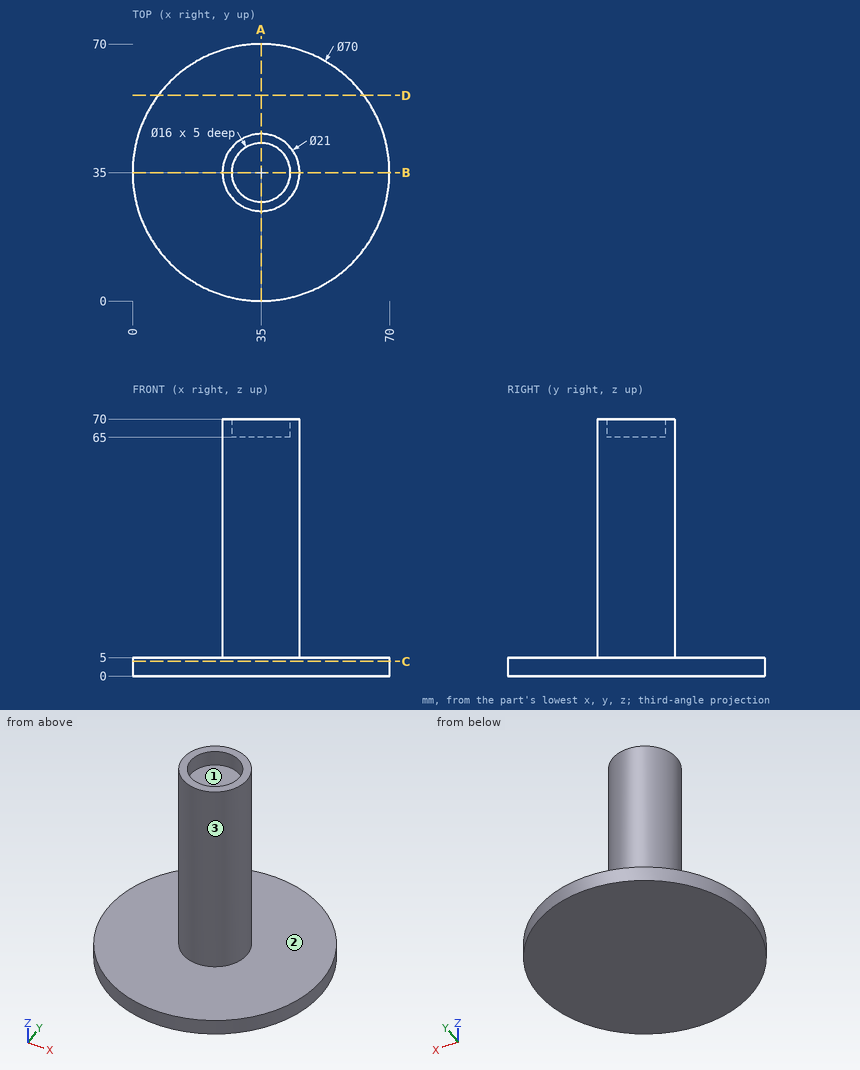
Verification items for this drawing (mm, ordinates from the low corner). Give positions to 0.01 mm unless a question says otherwise; leave off trailing zeros. Loops run counter-clockwise (first coordinate to the right, second up) from the corner with the lowest first, then second, coordinate; pieces in that order, holes last. Notation, with made-up numbers: M -37.75,-4 L -32.75,-4 A26 ccw -32.75,16 Z; hole C -38.5,87.25 d4. An arc over 180 degrees is marked long. Answer as CSV lines item,"result".
Item 1: Release check for a two-part mould opening along X. For the marked faces 1, 2 and 3 record: pulls with the +X half, pulls with the -X half, needs draft (parallel to the pull), parting line crosses it, or undercut.
Values:
face 1,"undercut"
face 2,"needs draft"
face 3,"parting line crosses it"
Item 2: Cross-section at D-D on y = 56. Record the cut outline in (x, z), and give its area (3 significant figures).
Values:
outline,"M 7,0 L 63,0 L 63,5 L 7,5 Z"
area,"280 mm²"
Item 3: Material ranges on line 1 (Y direction, x = 35, z = 68); line 2 (Z direction, x = 34, y = 50.5); line 3 (X direction, y = 37, z = 67), recorded low to high.
Values:
line 1,"y = 24.5 to 27, 43 to 45.5"
line 2,"z = 0 to 5"
line 3,"x = 24.69 to 27.25, 42.75 to 45.31"
Item 4: Cross-section at C-C on z = 4. Record the cut outline in (x, y), and give its area (3 significant figures).
Values:
outline,"C 35,35 d70"
area,"3,850 mm²"
Item 5: Depth check by flat-ended pin: P1, Ø6, axis at x = 19.5, z = 20.5, coming from the -Y side; P2, Ø3, axis at y = 39, z = 44.5, coming from the -X side; P3, Ø8, axis at x = 38, z = 54, coming from the -Y side; P4, Ø4, axis at x = 22.5, y = 11, coming from the +Z side. Enter the tip coordinate at first touch or a pass-through.
Values:
P1,"passes through"
P2,"stops at x = 24.8"
P3,"stops at y = 24.5"
P4,"stops at z = 5"
Item 6: Cross-section at A-A on x = 35. Record the cut outline in (y, z), and give its area (4 significant figures).
Values:
outline,"M 0,0 L 70,0 L 70,5 L 45.5,5 L 45.5,70 L 43,70 L 43,65 L 27,65 L 27,70 L 24.5,70 L 24.5,5 L 0,5 Z"
area,"1,635 mm²"
